For this review, take the finished solid that the model builds, in its own axes (mm). Coordinates: 2 decimals unless noted, no trailing zeros. Write each loop counter-clockwise with the first axis right and the second up, starting at its lowest first coordinate (ties: lowest second). Pieces come first, ordered by that corner, then holes. Notation, with made-up numbers: (14, 39.5) -> (57, 39.5) arc R29 ccw to (57, 69.5) -> close; hole circle Ø10 at (81.5, 1). An arc over 180 degrees is marked (long way). One line per item, written item: value. Start each with the question number.
1) Add section C-C (y = 5.25). State the section outline as (x, z) points, and give its area (3 significant figures).
2) Add section B-B (z = 0). State the section outline as (x, y) points.
3) For probe 1 along X at (y, z) = (7, 0); probe 2 along X at (y, z) = (8.25, 137), list the stretches that pass through material, from the lowest coordinate up. Write a range as from..to.
4) Add section D-D (z = -410.5). State the section outline as (x, y) points.
5) Mouldability with a two-part tool opening along Z and no side actions: class faces 1 (the cylindrical face through (462.126, 5.07, -457.099)), 2 (the cylindrical face through (190.764, 5.07, -60.075)), 3 (the cylindrical face through (457.099, 5.07, 462.126)) as released by +Z, released by -Z, zero draft, split by the parting line, or undercut.
6) For pin 1 Ø6 at (x, y) = (-455, 8) entering from -Z; pin 2 Ø2 at (y, z) = (2.5, -295.5) entering from -X; pin 3 Ø2 at (x, y) = (-468, 8.5) entering from -Z, all flat-tipped, find the tip position at first contact; note any pin that passes through.
7) Add section A-A (x = 0). State the section outline as (y, z) points, and give its area (3 significant figures).
from build123d import *

# Parameters (mm, degrees)
SKETCH1_W           = 1200
SKETCH1_H           = 1200
BOSS_EXTRUDE1_DEPTH = 10
SKETCH2_R           = 200
CUT_EXTRUDE1_DEPTH  = 11
SKETCH3_R           = 1053.62312192
SKETCH3_R_2         = 650
CUT_EXTRUDE2_DEPTH  = 11


with BuildPart() as part:
    # Sketch1 → Boss-Extrude1 (new body)
    with BuildSketch(Plane(origin=(0, 0, 0), x_dir=(1, 0, 0), z_dir=(0, 1, 0))):
        Rectangle(SKETCH1_W, SKETCH1_H)
    extrude(amount=BOSS_EXTRUDE1_DEPTH)

    # Sketch2 → Cut-Extrude1 (cut, through all)
    with BuildSketch(Plane(origin=(0, 10, 0), x_dir=(1, 0, 0), z_dir=(0, 1, 0))):
        Circle(SKETCH2_R)
    extrude(amount=-CUT_EXTRUDE1_DEPTH, mode=Mode.SUBTRACT)

    # Sketch3 → Cut-Extrude2 (cut, through all)
    with BuildSketch(Plane(origin=(0, 10, 0), x_dir=(1, 0, 0), z_dir=(0, 1, 0))):
        Circle(SKETCH3_R)
        Circle(SKETCH3_R_2, mode=Mode.SUBTRACT)
    extrude(amount=-CUT_EXTRUDE2_DEPTH, mode=Mode.SUBTRACT)


solid = part.part
Numbers:
1. outline: (-600, -250) arc R650 ccw to (-250, -600) -> (250, -600) arc R650 ccw to (600, -250) -> (600, 250) arc R650 ccw to (250, 600) -> (-250, 600) arc R650 ccw to (-600, 250) -> close; hole circle Ø400 at (0, 0)
1. area: 1,130,000 mm²
2. outline: (-600, 0) -> (-200, 0) -> (-200, 10) -> (-600, 10) -> close; (200, 0) -> (600, 0) -> (600, 10) -> (200, 10) -> close
3. probe 1: -600..-200, 200..600
3. probe 2: -600..-145.71, 145.71..600
4. outline: (-503.97, 0) -> (503.97, 0) -> (503.97, 10) -> (-503.97, 10) -> close
5. face 1: released by -Z
5. face 2: undercut
5. face 3: released by +Z
6. pin 1: z = -467.11
6. pin 2: x = -579.46
6. pin 3: z = -452.12
7. outline: (0, -600) -> (10, -600) -> (10, -200) -> (0, -200) -> close; (0, 200) -> (10, 200) -> (10, 600) -> (0, 600) -> close
7. area: 8,000 mm²
